```python
from build123d import *

# Parameters (mm, degrees)
BOSS_EXTRUDE1_DEPTH = 5
FILLET1_R           = 10


with BuildPart() as part:
    # Sketch1 → Boss-Extrude1 (new body)
    with BuildSketch(Plane(origin=(0, 0, 0), x_dir=(1, 0, 0), z_dir=(0, 1, 0))):
        with BuildLine():
            Line((40.301843205, 25), (110.301843205, 25))
            Line((110.301843205, 25), (200.301843205, 25))
            Line((200.301843205, 25), (200.301843205, 155))
            Line((200.301843205, 155), (110.301843205, 155))
            Line((110.301843205, 155), (40.301843205, 155))
            Line((40.301843205, 155), (40.301843205, 180.27466017))
            ThreePointArc((40.301843205, 180.27466017), (0.301843205, 90), (40.301843205, -0.27466017))
            Line((40.301843205, -0.27466017), (40.301843205, 25))
        make_face()
    extrude(amount=BOSS_EXTRUDE1_DEPTH)

    # Fillet1
    fillet1_edges = [part.edges().sort_by_distance(p)[0] for p in [
        (200.301843205, 2.5, -155),
        (200.301843205, 2.5, -25),
    ]]
    fillet(fillet1_edges, radius=FILLET1_R)


solid = part.part
```
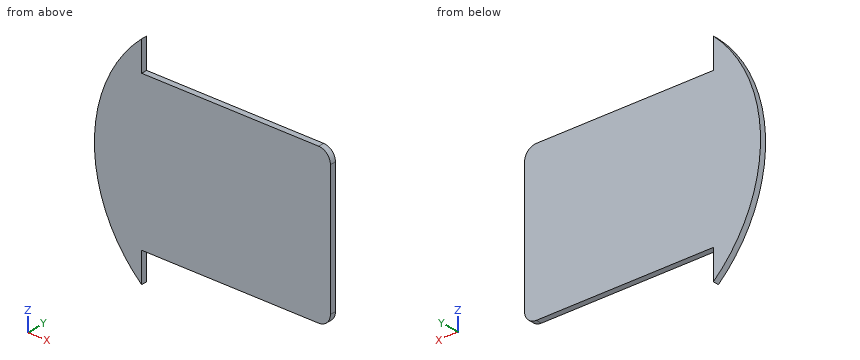
The listing builds one solid part. Answer for the finished solid, in the listing's coordinates (mm). Give positions to 0.01 mm unless a question says otherwise; leave off trailing zeros. Order: outer loops, then holes, each group sorted by start corner. A loop starts at its lowest first (then second) coordinate and runs counter-clockwise, first axis right, second up. Notation, with made-up numbers: (-18.5, 13) -> (2.5, 13) arc R14 ccw to (2.5, 20) -> close; hole circle Ø10 at (-39.5, 37.5). An arc over 180 degrees is marked (long way). Answer as a JSON object with one key per item and string values. Group by question number.
Item 1: Flat-ended cylindrical pins translate along their axes: pin 1 (3 mm diameter, centred on x = 23.5, y = 1.5, fed in from -Z); pin 2 (1.5 mm diameter, centred on y = 3, z = -171.5, fed in from +X); pin 3 (2 mm diameter, centred on x = 94.5, z = -23.5, fed in from +Y); pin 4 (1 mm diameter, centred on x = 66.5, y = 4, fed in from +Z). Find the tip coordinate at first contact, or state that the pin passes through.
Item 2: The part is cut by section A-A on y = 2.4. Write down the section's boundary in (x, z), and give its area (3 significant figures).
Item 3: The part is cut by section B-B on x = 67. Write down the section's boundary in (y, z), and give its area (3 significant figures).
Item 4: Consider L1, parallel to Z at x = 55, y = 2.05; L2, parallel to X at y = 3.8, z = -114; L3, parallel to X at y = 2.3, z = -87.5. Determine where each line is inside the solid, lowest interval first. Write a range as from..to.
Item 5: The part is cut by section C-C on z = -13. Write down the section's boundary in (x, y).
Result set:
{
 "1": {"pin 1": "z = -163.55", "pin 2": "x = 40.3", "pin 3": "through", "pin 4": "z = -25"},
 "2": {"outline": "(40.3, -180.27) -> (40.3, -155) -> (190.3, -155) arc R10 ccw to (200.3, -145) -> (200.3, -35) arc R10 ccw to (190.3, -25) -> (40.3, -25) -> (40.3, 0.27) arc R121.87 ccw to start", "area": "25,800 mm²"},
 "3": {"outline": "(0, -155) -> (5, -155) -> (5, -25) -> (0, -25) -> close", "area": "650 mm²"},
 "4": {"L1": "-155..-25", "L2": "2.69..200.3", "L3": "0.33..200.3"},
 "5": {"outline": "(27.71, 0) -> (40.3, 0) -> (40.3, 5) -> (27.71, 5) -> close"}
}
